Here's how the part is built. I have some questions about the finished solid (model axes, mm). Round coordinates to 2 decimals unless told otherwise and drop trailing zeros. Use one line per item in the form item = value. Start each with the question number.
Q1. I'm going to push flat-ended pins straight in: pin 1 Ø1 at (x, z) = (8, 1) entering from -Y; pin 2 Ø1 at (y, z) = (-24, 0.5) entering from -X; pin 3 Ø6 at (x, y) = (13, -16) entering from +Z; pin 4 Ø2 at (x, y) = (-14.53, -40.29) entering from +Z. Where does each tip first touch, or does it pass through?
Q2. I need wall thicknesses on line 1 along X through (y, z) = (-24, 1.85); line 2 along X through (y, z) = (-24, 1.1); line 3 along Y through (x, z) = (8, 1.15). Which ranges of each line are inside material? Lowest first, please. Write a range as from..to.
Q3. I want a section at D-D on z = 0.85. State how many separate pieces and enclosed holes the cut face has, and give its area (3 significant figures).
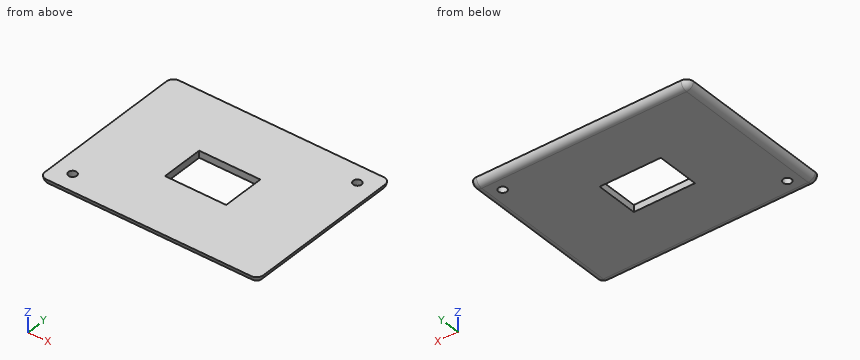
Autodesk Inventor part; units mm, degrees
ref_plane "YZ Plane" through (0, 0, 0) normal (1, 0, 0) x (0, 1, 0)
ref_plane "XZ Plane" through (0, 0, 0) normal (0, 1, 0) x (-1, 0, 0)
ref_plane "XY Plane" through (0, 0, 0) normal (0, 0, 1) x (1, 0, 0)
sketch "Sketch1" plane through (0, 0, 0) normal (0, 0, 1) x (1, 0, 0)
  line L0 (-19.8753, 2.5645) -> (43.3247, 2.5645)
  line L1 (43.3247, 2.5645) -> (43.3247, -45.6355)
  line L2 (43.3247, -45.6355) -> (-19.8753, -45.6355)
  line L3 (-19.8753, -45.6355) -> (-19.8753, 2.5645)
  circle A0 centre (37.9747, -2.7855) radius 2.1
  circle A1 centre (-14.5253, -40.2855) radius 2.1
  circle A2 centre (37.9747, -2.7855) radius 1.2
  circle A3 centre (-14.5253, -40.2855) radius 1.2
  point P0 (0, 0)
  dimension "d0" = 63.2
  dimension "d1" = 48.2
  dimension "d6" = 4.2
  dimension "d7" = 4.2
  dimension "d8" = 5.35
  dimension "d9" = 5.35
  dimension "d10" = 5.35
  dimension "d11" = 5.35
  dimension "d12" = 2.4
  dimension "d13" = 2.4
extrude "Extrusion1" add sketch "Sketch1" along normal blind 2 contours L0 L1 L2 L3 | A0 | A1 | A2 | A3
fillet "Fillet1" radius 2 2 edges at (-19.8753, 2.5645, 1) (-19.8753, -45.6355, 1)
fillet "Fillet2" radius 2 2 edges at (43.3247, 2.5645, 1) (43.3247, -45.6355, 1)
sketch "Sketch2" plane through (0, 0, 0) normal (0, 0, -1) x (-1, 0, 0)
  circle A0 centre (14.5253, -40.2855) radius 2.1
  circle A1 centre (-37.9747, -2.7855) radius 2.1
  circle A2 centre (14.5253, -40.2855) radius 1.2
  circle A3 centre (-37.9747, -2.7855) radius 1.2
  line L0 (17.8753, -45.6355) -> (-41.3247, -45.6355)
  line L1 (19.8753, 0.5645) -> (19.8753, -43.6355)
  line L2 (-43.3247, -43.6355) -> (-43.3247, 0.5645)
  line L3 (-41.3247, 2.5645) -> (17.8753, 2.5645)
  point P0 (0, 0)
  dimension "d14" = 4.2
  dimension "d15" = 4.2
  dimension "d16" = 2.4
  dimension "d17" = 2.4
  dimension "d18" = 5.35
  dimension "d19" = 5.35
  dimension "d20" = 5.35
  dimension "d21" = 5.35
extrude "Extrusion3" cut sketch "Sketch2" against normal blind 2.2 contours A2 | A3
fillet "Fillet3" radius 2 8 edges at (42.7389, -45.0497, 0) (43.3247, -21.5355, 0) (42.7389, 1.9787, 0) (11.7247, 2.5645, 0) (-19.2896, 1.9787, 0) (-19.8753, -21.5355, 0) (-19.2896, -45.0497, 0) (11.7247, -45.6355, 0)
sketch "Sketch4" plane through (0, 0, 0) normal (0, 0, -1) x (-1, 0, 0)
  line L0 (-2.3639, -27.9277) -> (-20.0539, -27.9277)
  line L1 (-20.0539, -27.9277) -> (-20.0539, -15.5277)
  line L2 (-20.0539, -15.5277) -> (-2.3639, -15.5277)
  line L3 (-2.3639, -15.5277) -> (-2.3639, -27.9277)
  point P0 (0, 0)
  dimension "d27" = 17.69
  dimension "d28" = 12.4
extrude "Extrusion4" cut sketch "Sketch4" against normal blind 2.2
properties part number "limb_cover"
Reported:
q1.pin_1 = -45.57
q1.pin_2 = -19.61
q1.pin_3 = 2
q1.pin_4 = through
q2.line_1 = -19.87..2.36, 20.05..43.32
q2.line_2 = -19.66..2.36, 20.05..43.11
q2.line_3 = -45.45..-27.93, -15.53..2.38
q3.separate_pieces = 1
q3.enclosed_holes = 3
q3.area = 2,740 mm^2
